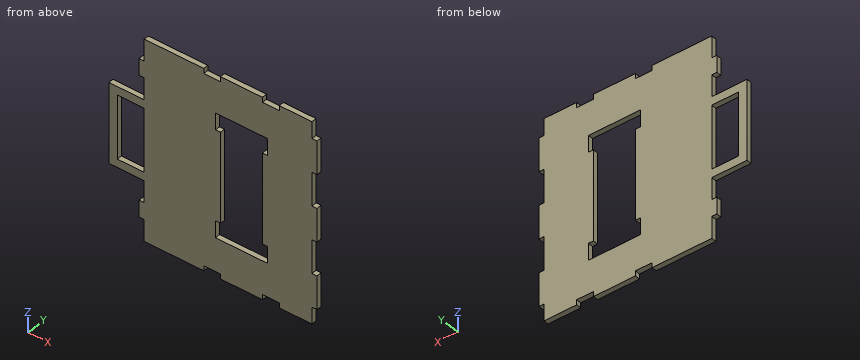
Autodesk Inventor part; units mm, degrees
ref_plane "YZ Plane" through (0, 0, 0) normal (1, 0, 0) x (0, 1, 0)
ref_plane "XZ Plane" through (0, 0, 0) normal (0, 1, 0) x (-1, 0, 0)
ref_plane "XY Plane" through (0, 0, 0) normal (0, 0, 1) x (1, 0, 0)
sketch "Sketch1" plane through (0, 0, 0) normal (0, 1, 0) x (-1, 0, 0)
  line L0 (50, 60) -> (-50, 60)
  line L1 (-50, 60) -> (-50, -60)
  line L2 (-50, -60) -> (50, -60)
  line L3 (50, -60) -> (50, 60)
  line L4 (50, 60) -> (-50, -60) construction
  line L5 (-50, 60) -> (50, -60) construction
  point P0 (0, 0)
  dimension "d0" = 60
  dimension "d1" = 100
extrude "Extrusion1" add sketch "Sketch1" along normal blind 3
sketch "Sketch2" plane through (0, 3, 0) normal (0, 1, 0) x (1, 0, 0)
  line L0 (-50, -60) -> (50, -60)
  line L1 (-14.5, -60) -> (-4.5, -60)
  line L2 (-4.5, -60) -> (-4.5, -57)
  line L3 (-4.5, -57) -> (-14.5, -57)
  line L4 (-14.5, -57) -> (-14.5, -60)
  line L5 (50, -60) -> (50, 60)
  line L6 (20.5, -60) -> (30.5, -60)
  line L7 (30.5, -60) -> (30.5, -57)
  line L8 (30.5, -57) -> (20.5, -57)
  line L9 (20.5, -57) -> (20.5, -60)
  line L10 (-4.5, -37) -> (-7.5, -37)
  line L11 (-7.5, -37) -> (-7.5, -27)
  line L12 (-7.5, -27) -> (-4.5, -27)
  line L13 (-4.5, -27) -> (-4.5, -37)
  line L14 (20.5, -27) -> (23.5, -27)
  line L15 (23.5, -27) -> (23.5, -37)
  line L16 (23.5, -37) -> (20.5, -37)
  line L17 (20.5, -37) -> (20.5, -27)
  point P0 (0, 0)
  dimension "d4" = 10
  dimension "d5" = 3
  dimension "d6" = 54.5
  dimension "d7" = 10
  dimension "d8" = 3
  dimension "d9" = 25
  dimension "d10" = 3
  dimension "d11" = 10
  dimension "d12" = 30
  dimension "d13" = 3
  dimension "d14" = 10
extrude "Extrusion2" cut sketch "Sketch2" against normal blind 3
sketch "Sketch3" plane through (0, 3, 0) normal (0, 1, 0) x (1, 0, 0)
  line L0 (50, -60) -> (50, 60)
  line L1 (50, 10) -> (53, 10)
  line L2 (53, 10) -> (53, -10)
  line L3 (53, -10) -> (50, -10)
  line L4 (50, -10) -> (50, 10)
  line L5 (50, -30) -> (53, -30)
  line L6 (53, -30) -> (53, -50)
  line L7 (53, -50) -> (50, -50)
  line L8 (50, -50) -> (50, -30)
  line L9 (50, 30) -> (53, 30)
  line L10 (53, 30) -> (53, 50)
  line L11 (53, 50) -> (50, 50)
  line L12 (50, 50) -> (50, 30)
  point P0 (0, 0)
  point P1 (53, 0)
  dimension "d17" = 3
  dimension "d18" = 20
  dimension "d19" = 3
  dimension "d20" = 20
  dimension "d21" = 20
  dimension "d22" = 20
extrude "Extrusion3" add sketch "Sketch3" against normal blind 3
sketch "Sketch4" plane through (0, 3, 0) normal (0, 1, 0) x (1, 0, 0)
  line L0 (-50, 60) -> (-50, -60)
  line L1 (-50, 24) -> (-71, 24)
  line L2 (-71, 24) -> (-71, -24)
  line L3 (-71, -24) -> (-50, -24)
  line L4 (-50, -24) -> (-50, 24)
  line L5 (-50, -19) -> (-66, -19)
  line L6 (-66, -19) -> (-66, 19)
  line L7 (-66, 19) -> (-50, 19)
  line L8 (-50, 19) -> (-50, -19)
  point P0 (0, 0)
  point P1 (-71, 0)
  point P2 (-66, 0)
  dimension "d27" = 38
  dimension "d28" = 16
  dimension "d29" = 5
  dimension "d30" = 5
extrude "Extrusion4" add sketch "Sketch4" against normal blind 3 contours L0 L7 L6 L5 L3 L2 L1
sketch "Sketch6" plane through (0, 3, 0) normal (0, 1, 0) x (1, 0, 0)
  line L0 (-50, 60) -> (-50, 24)
  line L1 (-50, 47) -> (-53, 47)
  line L2 (-53, 47) -> (-53, 37)
  line L3 (-53, 37) -> (-50, 37)
  line L4 (-50, 37) -> (-50, 47)
  line L5 (-50, 24) -> (-71, 24)
  point P0 (0, 0)
  dimension "d39" = 3
  dimension "d40" = 10
  dimension "d41" = 13
  dimension "d42" = 13
extrude "Extrusion6" add sketch "Sketch6" against normal blind 3
sketch "Sketch8" plane through (0, 3, 0) normal (0, 1, 0) x (1, 0, 0)
  line L0 (20.5, -37) -> (-4.5, -37)
  line L1 (-4.5, -37) -> (-4.5, 37)
  line L2 (-4.5, 37) -> (20.5, 37)
  line L3 (20.5, 37) -> (20.5, -37)
  line L4 (-4.5, -27) -> (-4.5, -37)
  point P0 (0, 0)
  point P1 (20.5, 0)
extrude "Extrusion7" cut sketch "Sketch8" against normal blind 3
mirror "Mirror1" about plane through (0, 0, 0) normal (0, 0, 1) of "Extrusion2"
mirror "Mirror2" about plane through (0, 0, 0) normal (0, 0, 1) of "Extrusion6"
equation "\"d30\" = d29"
equation "\"d41\" = d42"
properties part number "Mid Plate"
CAD build for the part. Positions are in the model's coordinates, mm. Give positions to 0.01 mm unless a question says otherwise; leave off trailing zeros. Order: outer loops, then holes, each group sorted by start corner. A loop starts at its lowest first (then second) coordinate and runs counter-clockwise, first axis right, second up. Notation, with made-up numbers: M -8,81.5 L 20,81.5 A13 cw 20,101.5 Z; hole C 76.25,45 d10. An arc over 180 degrees is marked long. Put each result on its own line as item: value. Start each with the question number.
(1) Flat gauge pins, fed straight in: pin 1 Ø1.5 at (y, z) = (1, -58) entering from +X; pin 2 Ø0.9 at (y, z) = (2, -58) entering from -X; pin 3 Ø1.5 at (x, y) = (51, 1) entering from +Z. Where does each tip first touch, or does it go through?
(2) Saw through at B-B, the plane x = -1. Write the cut outline in (y, z).
(3) Saw through at D-D, the plane x = -61. Write the cut outline in (y, z).
(4) Saw through at A-A, the plane z = -16. Write the cut outline in (x, y), then the cut area to 3 significant figures.
(5) Drill centre lines: line 1 along X through (y, z) = (1.6, 6); line 2 along Z through (x, y) = (22.5, 1.75); line 3 along X through (y, z) = (1.1, 36.5). Where is each one in solid material? Low to high.
(6) Saw through at C-C, the plane z = -2. Write the cut outline in (x, y).
Check result:
1. pin 1: stops at x = 50
1. pin 2: stops at x = -50
1. pin 3: stops at z = 50
2. outline: M 0,-60 L 3,-60 L 3,-37 L 0,-37 Z; M 0,37 L 3,37 L 3,60 L 0,60 Z
3. outline: M 0,-24 L 3,-24 L 3,-19 L 0,-19 Z; M 0,19 L 3,19 L 3,24 L 0,24 Z
4. outline: M -71,0 L -66,0 L -66,3 L -71,3 Z; M -50,0 L -4.5,0 L -4.5,3 L -50,3 Z; M 20.5,0 L 50,0 L 50,3 L 20.5,3 Z
4. area: 240 mm2
5. line 1: x = -71 to -66, -50 to -4.5, 20.5 to 53
5. line 2: z = -57 to -37, -27 to 27, 37 to 57
5. line 3: x = -50 to -7.5, 23.5 to 53
6. outline: M -71,0 L -66,0 L -66,3 L -71,3 Z; M -50,0 L -4.5,0 L -4.5,3 L -50,3 Z; M 20.5,0 L 53,0 L 53,3 L 20.5,3 Z
